Part print with two shaded views. Sizes in mm from the minimum x, y, z corner. A direction names the side the tool comes from. Coordinates: 2 decimals unless noted, no trailing zeros. Order: outer loops, then holes, each group sorted by start corner. A loop starts at its lowest first (then second) coordinate and runs counter-clockwise, first axis right, second up. Notation, with made-up numbers: (34, 46.25) - (58, 46.25) arc R19 cw to (58, 52.25) - close; hole circle Ø8 at (-20.75, 9.25). An arc over 180 degrees is marked (long way). Return JSON: item names as keys, results as strings.
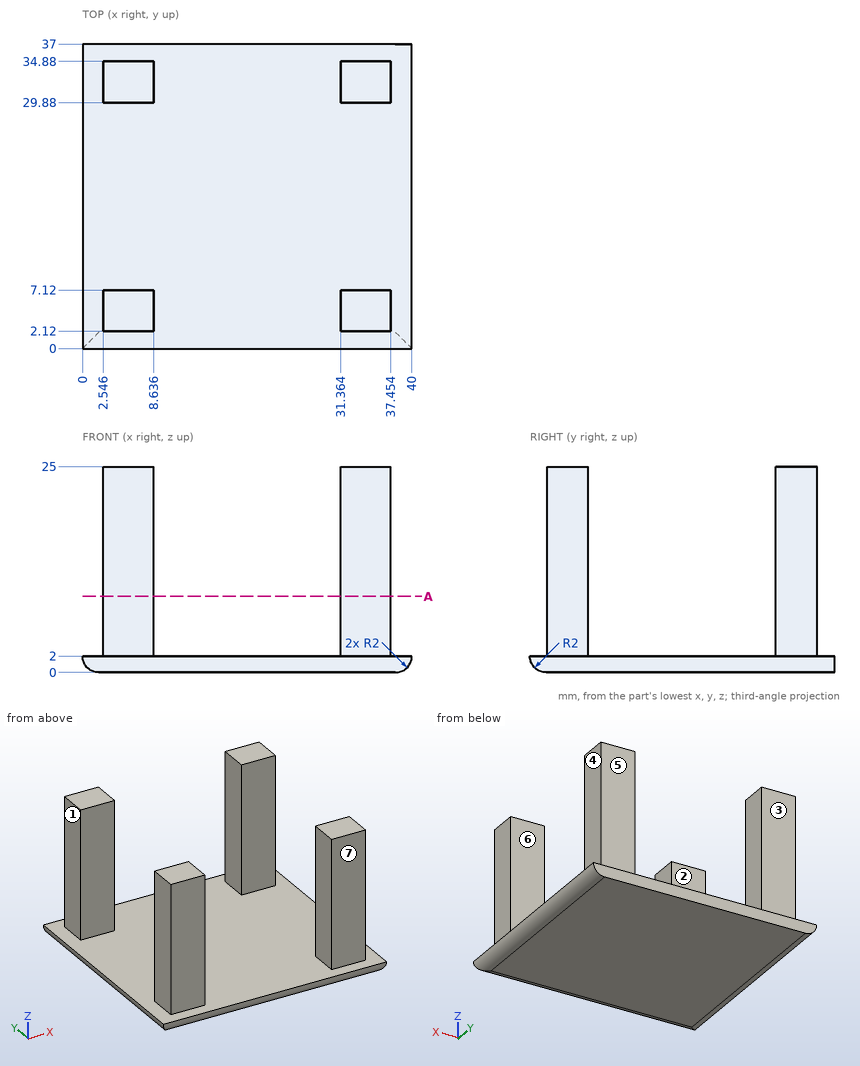
Item 1: Mould opens along Y. For the marked faces 4, 5, 6 and 7 say: released by +Y, released by -Y, zero draft, split by the parting line, or undercut.
Findings below:
{"face 4": "zero draft", "face 5": "released by +Y", "face 6": "undercut", "face 7": "released by -Y"}
Item 2: Wall check: L1, parallel to X at y = 3.5, z = 23.5 (1 decimal); L2, parallel to Y at x = 36.5, z = 3; L3, parallel to Z at x = 36, y = 21. Give the ranges that are in metal, low to high. Write a range as [from, to].
Findings below:
{"L1": "x = [2.5, 8.6], [31.4, 37.5]", "L2": "y = [2.12, 7.12], [29.88, 34.88]", "L3": "z = [0, 2]"}
Item 3: Band-saw the part on A-A, the plane z = 9.25. List the corners of the cut face in (x, y) (1 decimal), then the cut area to 3 significant figures.
Findings below:
{"outline": "(2.5, 2.1) - (8.6, 2.1) - (8.6, 7.1) - (2.5, 7.1) - close; (2.5, 29.9) - (8.6, 29.9) - (8.6, 34.9) - (2.5, 34.9) - close; (31.4, 2.1) - (37.5, 2.1) - (37.5, 7.1) - (31.4, 7.1) - close; (31.4, 29.9) - (37.5, 29.9) - (37.5, 34.9) - (31.4, 34.9) - close", "area": "122 mm²"}
Item 4: Which spindle directions (+Z, -Z, +X, -X, +Y, -Y) get a long thin tool onto all of the face, cutting with end or side? Do the marked faces 1, 2 and 3. Say none if no direction does.
Findings below:
{"face 1": "+Z, -X, +Y, -Y", "face 2": "+Z, +X, -X", "face 3": "+Z, +X, -X, +Y"}
Item 5: Drop flat-ended pins along their axis: P1, Ø11, axis at x = 25, y = 20.5, coming from the +Z side; P2, Ø1.5, axis at y = 31.5, z = 12.5, coming from the -X side (1 decimal); P3, Ø2.5, axis at y = 32.5, z = 13.5, coming from the +X side (1 decimal); P4, Ø12, axis at x = 10, y = 12.5, coming from the -Z side. Give the stop position or say it passes through.
Findings below:
{"P1": "stops at z = 2", "P2": "stops at x = 2.5", "P3": "stops at x = 37.5", "P4": "stops at z = 0"}
